Geometry check sheet. Reference: the model listing, model coordinates, mm. A direction names the side the tool comes from. Coordinates: 2 decimals unless noted, no trailing zeros. Loops run counter-clockwise (first coordinate to the right, second up) from the corner with the lowest first, then second, coordinate; pieces in that order, holes last. Notation, with made-up numbers: M -32,75 L -22,75 A26 cw -22,98 Z; hole C 50.5,56 d2. An arc over 180 degrees is marked long. Use CSV: the item, a comma, the result in double quotes.
```python
from build123d import *

# Parameters (mm, degrees)
F0_R     = 29.21
F1_DEPTH = 13.462
F2_R     = 1.778
F3_DEPTH = 2.54


# Not quite as in the source:
# - a pattern or mirror of a feature is missing from the dataset's text; its kind, count and spacing are read off the source's solid


with BuildPart() as f1:
    # F0 (on Top) → F1 (new body, symmetric)
    with BuildSketch(Plane.XY):
        Circle(F0_R)
    extrude(amount=F1_DEPTH, both=True)

    # F2 (on face) → F3 (cut)
    with BuildSketch(Plane.XY.offset(13.462)):
        Circle(F2_R)
    f3 = extrude(amount=-F3_DEPTH, mode=Mode.SUBTRACT)

    # F3_copies: F3 across plane
    add(f3.mirror(Plane(origin=(0, 0, 0), x_dir=(-1, 0, 0), z_dir=(0, 0, -1))), mode=Mode.SUBTRACT)


solid = f1.part
```
1. Gauge pin test, flat ends, axial feed: P1, Ø1.5, axis at y = -14.5, z = 6, coming from the -X side; P2, Ø3, axis at x = 0, y = 0, coming from the +Z side; P3, Ø2, axis at x = 6.5, z = -9, coming from the +Y side. Record the tip position at first contact, or that the pin passes through.
The answers:
P1,"x = -25.77"
P2,"z = 10.92"
P3,"y = 28.69"
2. Section check A-A, the plane y = -6.5. Record the cut outline in (x, z), plus the area to 3 significant figures.
The answers:
outline,"M -28.48,-13.46 L 28.48,-13.46 L 28.48,13.46 L -28.48,13.46 Z"
area,"1,530 mm^2"
3. Release check for a two-part mould opening along Y. For faces 1 (the flat face through (0, -6, 13.462)), 2 (the cylindrical face through (-21.53, 19.74, 0.19)), 3 (the cylindrical face through (-0.385, -1.736, 12.21)) record: +Y half, -Y half, draft (parallel to the pull), parting line (faces both ways), or undercut.
The answers:
face 1,"draft"
face 2,"parting line"
face 3,"undercut"
4. Set-up check for faces 4 (the flat face through (0, 0, -10.922)), 5 (the flat face through (0, 0, 10.922)), 6 (the flat face through (0, -6, -13.462)): record each of +Z, -Z, +X, -X, +Y, -Y from which the full face is reachable in a straight line by a thin tool's end or side.
The answers:
face 4,"-Z"
face 5,"+Z"
face 6,"-Z, +X, -X, +Y, -Y"
5. Thickness scan on line 1 (Y direction, x = 0, z = 12.45); line 2 (Z direction, x = 0, y = 1.5); line 3 (X direction, y = 22, z = 8.75). Record the ranges inside material, lowest first. Write a range as [from, to].
The answers:
line 1,"[-29.21, -1.78], [1.78, 29.21]"
line 2,"[-10.92, 10.92]"
line 3,"[-19.22, 19.22]"
6. Section check B-B, the plane x = -11.5. Record the cut outline in (y, z).
The answers:
outline,"M -26.85,-13.46 L 26.85,-13.46 L 26.85,13.46 L -26.85,13.46 Z"
7. Section check C-C, the plane z = -5.5. Record the cut outline in (x, y).
The answers:
outline,"C 0,0 d58.42"
